from build123d import *

# Parameters (mm, degrees)
BOSS_EXTRUDE1_DEPTH = 12.25
SKETCH2_W           = 84.1
SKETCH2_H           = 6.35
BOSS_EXTRUDE2_DEPTH = 10
FILLET1_R           = 1


with BuildPart() as part:
    # Sketch1 → Boss-Extrude1 (new body)
    with BuildSketch(Plane(origin=(0, 0, 0), x_dir=(1, 0, 0), z_dir=(0, 1, 0))):
        with BuildLine():
            Line((17.364817767, 98.480775301), (46.909050357, 93.271329971))
            Line((46.909050357, 93.271329971), (98.097719862, 22.625355106))
            ThreePointArc((98.097719862, 22.625355106), (99.512549569, 19.841964096), (100, 16.757908213))
            Line((100, 16.757908213), (100, 10))
            ThreePointArc((100, 10), (97.071067812, 2.928932188), (90, 0))
            Line((90, 0), (70, 0))
            Line((70, 0), (1.736481777, 9.84807753))
            Line((1.736481777, 9.84807753), (17.364817767, 98.480775301))
        make_face()
        Polygon((40.041775538, 82.297096463), (88, 16.109489855), (88, 12), (70.861136072, 12), (15.704122693, 19.957259723), (27.098732671, 84.579304133), align=None, mode=Mode.SUBTRACT)
    extrude(amount=BOSS_EXTRUDE1_DEPTH)

    # Sketch2 → Boss-Extrude2 (add)
    with BuildSketch(Plane(origin=(0, 0, 0), x_dir=(-0.17364817766692336, 0, 0.9848077530122094), z_dir=(-0.9848077530122092, 0, -0.17364817766692334))):
        with Locations((-55, 6.125)):
            Rectangle(SKETCH2_W, SKETCH2_H)
    extrude(amount=BOSS_EXTRUDE2_DEPTH)

    # Fillet1
    fillet1_edges = [part.edges().sort_by_distance(p)[0] for p in [
        (-0.297427758, 2.95, -55.900908192),
        (-7.599333629, 6.125, -14.489742178),
        (-0.297427758, 9.3, -55.900908192),
        (7.004478112, 6.125, -97.312074207),
    ]]
    fillet(fillet1_edges, radius=FILLET1_R)


solid = part.part
Work out the finished part from the listing and answer in its coordinate system (mm). A direction names the side the tool comes from. Round coordinates to 2 decimals unless told otherwise and drop trailing zeros. Order: outer loops, then holes, each group sorted by start corner. A loop starts at its lowest first (then second) coordinate and runs counter-clockwise, first axis right, second up. Notation, with made-up numbers: M 80.5,89 L 124.5,89 A17 cw 124.5,93 Z; hole C 38.25,8 d1. An arc over 180 degrees is marked long. Put each result on its own line as item: value. Start each with the question number.
Q1. For a pull along Z with two mould halves and no side action, classify faces 1 (the flat face through (80, 6, 0)), 2 (the flat face through (31.93, 6.039, -95.913)), 3 (the flat face through (66, 0, -49)), 4 (the flat face through (63.685, 6.039, -49.667)) as pulls with the +Z half, pulls with the -Z half, needs draft (parallel to the pull), parting line crosses it, or undercut.
Q2. Straight lines are drawn through the part: L1, parallel to Y at x = 4, z = -41; L2, parallel to Z at x = 54.5, y = 4.25. For each, find the intervals that lie inside material, in ascending order. Write a range as [from, to].
Q3. Flat-ended cylindrical pins translate along their axes: pin 1 (1 mm diameter, centred on x = 60, y = 1.5, fed in from +Z); pin 2 (6 mm diameter, centred on y = 9, z = -20, fed in from +X); pin 3 (4 mm diameter, centred on x = 5.5, y = 10, fed in from +Z); pin 4 (10 mm diameter, centred on x = 29.5, z = -51, fed in from +Y). Find the tip coordinate at first contact, or state that the pin passes through.
Q4. Section A-A, the plane y = 7 is taken. Write down the section's boundary in (x, z).
Q5. Section C-C, the plane x = 63 is taken. Write down the section's boundary in (y, z).
Q6. A tool of negligible diameter and unlimited length cuts with its end or side. For faces 5 (the flat face through (5, 2.95, -56)), 6 (the flat face through (88, 6, -14)), 7 (the flat face through (36.346, 6.039, -4.855)), 8 (the flat face through (100, 6, -13)), 9 (the flat face through (5, 9.3, -56)), from which of +Z, -Z, +X, -X, +Y, -Y can it reach the whole face along a straight path? Write none if from no direction.
Q7. Section B-B, the plane x = 42 is taken. Write down the section's boundary in (y, z), and give its area (3 significant figures).
Findings below:
1. face 1: pulls with the +Z half
1. face 2: pulls with the -Z half
1. face 3: needs draft
1. face 4: undercut
2. L1: y = [2.95, 9.3]
2. L2: z = [-82.79, -62.34], [-14.36, -2.24]
3. pin 1: stops at z = -1.37
3. pin 2: stops at x = 100
3. pin 3: stops at z = -9.02
3. pin 4: passes through
4. outline: M -7.43,-15.47 L 6.83,-96.33 A1 ccw 7.99,-97.14 L 16.85,-95.58 L 17.36,-98.48 L 46.91,-93.27 L 98.1,-22.63 A10 ccw 100,-16.76 L 100,-10 A10 ccw 90,0 L 70,0 L 1.74,-9.85 L 2.25,-12.75 L -6.61,-14.32 A1 ccw Z; hole M 15.7,-19.96 L 27.1,-84.58 L 40.04,-82.3 L 88,-16.11 L 88,-12 L 70.86,-12 Z
5. outline: M 0,-71.06 L 12.25,-71.06 L 12.25,-50.61 L 0,-50.61 Z; M 0,-13.13 L 12.25,-13.13 L 12.25,-1.01 L 0,-1.01 Z
6. face 5: -Z, -X, -Y
6. face 6: +Y, -Y
6. face 7: +Z, -X, +Y, -Y
6. face 8: +Z, -Z, +X, +Y, -Y
6. face 9: -Z, -X, +Y
7. outline: M 0,-94.14 L 12.25,-94.14 L 12.25,-79.59 L 0,-79.59 Z; M 0,-16.16 L 12.25,-16.16 L 12.25,-4.04 L 0,-4.04 Z
7. area: 327 mm^2
